Could you check a few things on this drawing? It's one solid part, dimensions in mm from its lowest x, y, z. A direction names the side the tool comes from. Round coordinates to 2 decimals unless told otherwise and drop trailing zeros. Loops run counter-clockwise (first coordinate to the right, second up) from the corner with the lowest first, then second, coordinate; pieces in that order, holes last. Notation, with made-up numbers: (29.25, 68) -> (66.25, 68) arc R22 ccw to (66.25, 84) -> close; hole circle Ø4 at (56.25, 2.5). An arc over 180 degrees is marked (long way). Put each result on its own line as item: value. Start each with the question number.
1. Imagine slicing it at B-B, the plane z = 0.6. Please give me the cut outline in (x, y).
2. I'm going to push a flat-ended pin straight in: P1, Ø5, axis at x = 7, y = 10, coming from the +Z side. Where does the tip first touch, or does it pass through?
3. If we mould it in two halves opening along Y, with no side actions, what happens to the marked faces 3, 4 and 5? For each: pulls with the +Y half, pulls with the -Y half, needs draft (parallel to the pull), parting line crosses it, or undercut.
4. I need wall thicknesses on line 1 (X direction, y = 6.5, z = 3.5); line 2 (X direction, y = 5, z = 4.8); line 3 (Y direction, x = 4, z = 4.8) (1 decimal). Which ranges of each line are inside material? Lowest first, please. Write a range as [from, to].
5. Imagine slicing it at C-C, the plane x = 5.5. Please give me the cut outline in (y, z) (1 decimal).
6. Imagine slicing it at D-D, the plane y = 1.75. Please give me the cut outline in (x, z).
7. Which directions (+Z, -Z, +X, -X, +Y, -Y) give clear straight access to the entire face, cutting with the end or side of a thin tool? Please do the marked faces 1 and 2.
8. Imagine slicing it at A-A, the plane y = 4. Please give me the cut outline in (x, z).
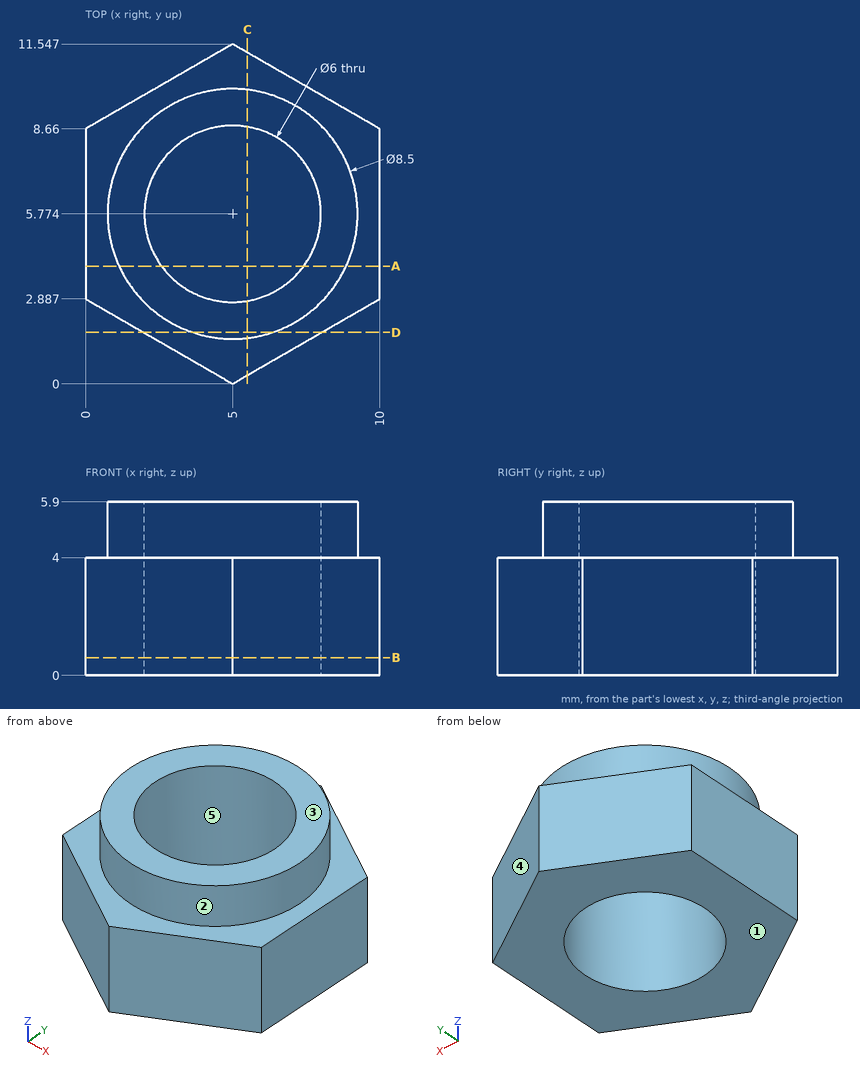
Entries:
1. outline: (0, 2.89) -> (5, 0) -> (10, 2.89) -> (10, 8.66) -> (5, 11.55) -> (0, 8.66) -> close; hole circle Ø6 at (5, 5.77)
2. P1: z = 5.9
3. face 3: needs draft
3. face 4: pulls with the +Y half
3. face 5: undercut
4. line 1: [0, 2.09], [7.91, 10]
4. line 2: [0.82, 2.1], [7.9, 9.18]
4. line 3: [1.6, 2.9], [8.6, 9.9]
5. outline: (0.3, 0) -> (2.8, 0) -> (2.8, 5.9) -> (1.6, 5.9) -> (1.6, 4) -> (0.3, 4) -> close; (8.7, 0) -> (11.3, 0) -> (11.3, 4) -> (10, 4) -> (10, 5.9) -> (8.7, 5.9) -> close
6. outline: (1.97, 0) -> (8.03, 0) -> (8.03, 4) -> (6.37, 4) -> (6.37, 5.9) -> (3.63, 5.9) -> (3.63, 4) -> (1.97, 4) -> close
7. face 1: -Z, +X, -X, +Y, -Y
7. face 2: +Z
8. outline: (0, 0) -> (2.58, 0) -> (2.58, 5.9) -> (1.14, 5.9) -> (1.14, 4) -> (0, 4) -> close; (7.42, 0) -> (10, 0) -> (10, 4) -> (8.86, 4) -> (8.86, 5.9) -> (7.42, 5.9) -> close
